Work out the finished part from the listing and answer in its coordinate system (mm). A direction names the side the tool comes from. Round coordinates to 2 decimals unless told otherwise and drop trailing zeros. Order: outer loops, then holes, each group sorted by start corner. A loop starts at its lowest first (then second) coordinate and runs counter-clockwise, first axis right, second up. Notation, with made-up numbers: M -25,80 L 8,80 A27 cw 8,113 Z; hole C -23.5,3.25 d9. An arc over 180 degrees is marked long. Return JSON: item names as keys, results as strings.
from build123d import *

# Parameters (mm, degrees)
BOSS_EXTRUDE1_DEPTH      = 10
BOSS_EXTRUDE1_DEPTH_BACK = 0.01
SKETCH1_W                = 98
SKETCH1_H                = 42
SKETCH1_R                = 6
FILLET1_R                = 5
FILLET2_R                = 5
SKETCH3_W                = 14
SKETCH3_H                = 42
BOSS_EXTRUDE4_DEPTH      = 10
SKETCH10_W               = 14
SKETCH10_H               = 42
BOSS_EXTRUDE5_DEPTH      = 10
SKETCH11_W               = 14
SKETCH11_H               = 42
BOSS_EXTRUDE6_DEPTH      = 42
FILLET3_RADIUS           = 21
FILLET3_LENGTH           = 14
CUT_EXTRUDE1_DEPTH       = 80.252760204
CUT_EXTRUDE1_DEPTH_BACK  = 80.252760204
SKETCH12_R               = 10


with BuildPart() as part:
    # Sketch1 → Boss-Extrude1 (new, two sides: drawn at the far end of the back side and taken through both)
    with BuildSketch(Plane(origin=(0, 0, 0), x_dir=(1, 0, 0), z_dir=(0, 1, 0)).offset(-BOSS_EXTRUDE1_DEPTH_BACK)):
        Rectangle(SKETCH1_W, SKETCH1_H)
        with Locations(Location((25, 0, 0), (0, 0, 270))):
            Circle(SKETCH1_R, mode=Mode.SUBTRACT)
        with Locations(Location((-25, 0, 0), (0, 0, 270))):
            Circle(SKETCH1_R, mode=Mode.SUBTRACT)
    extrude(amount=BOSS_EXTRUDE1_DEPTH + BOSS_EXTRUDE1_DEPTH_BACK)

    # Fillet1
    fillet1_edges = [part.edges().sort_by_distance(p)[0] for p in [
        (-49, 10, 0),
    ]]
    fillet(fillet1_edges, radius=FILLET1_R)

    # Fillet2
    fillet2_edges = [part.edges().sort_by_distance(p)[0] for p in [
        (49, 10, 0),
    ]]
    fillet(fillet2_edges, radius=FILLET2_R)

    # Sketch3 → Boss-Extrude4 (add)
    with BuildSketch(Plane.XZ.offset(0.01)):
        with Locations((-42, 0)):
            Rectangle(SKETCH3_W, SKETCH3_H)
    extrude(amount=BOSS_EXTRUDE4_DEPTH)

    # Sketch10 → Boss-Extrude5 (add)
    with BuildSketch(Plane.XZ.offset(0.01)):
        with Locations((42, 0)):
            Rectangle(SKETCH10_W, SKETCH10_H)
    extrude(amount=BOSS_EXTRUDE5_DEPTH)

    # Sketch11 → Boss-Extrude6 (add)
    with BuildSketch(Plane(origin=(0, 10, 0), x_dir=(1, 0, 0), z_dir=(0, 1, 0))):
        Rectangle(SKETCH11_W, SKETCH11_H)
    extrude(amount=BOSS_EXTRUDE6_DEPTH)

    # Fillet3: full round fillet: the end face becomes a half cylinder, R = half its width
    fillet3_face = Plane((0, 52, 0), x_dir=(1, 0, 0), z_dir=(0, 1, 0))  # on the end face: x along it, z out of the body
    fillet3_slab = fillet3_face.offset(-FILLET3_RADIUS / 2) * Box(FILLET3_LENGTH, 2 * FILLET3_RADIUS, FILLET3_RADIUS, mode=Mode.PRIVATE)  # the body's end, R deep
    fillet3_round = Plane((0, 31, 0), x_dir=(0, 1, 0), z_dir=(1, 0, 0)) * Cylinder(FILLET3_RADIUS, FILLET3_LENGTH, mode=Mode.PRIVATE)  # its axis R under the face
    add(fillet3_slab - fillet3_round, mode=Mode.SUBTRACT)

    # Sketch12 → Cut-Extrude1 (cut, two sides: drawn at the far end of the back side and taken through both)
    with BuildSketch(Plane(origin=(7, 0, 0), x_dir=(0, 0, -1), z_dir=(1, 0, 0)).offset(-CUT_EXTRUDE1_DEPTH_BACK)):
        with Locations((0, 31)):
            Circle(SKETCH12_R)
    extrude(amount=CUT_EXTRUDE1_DEPTH + CUT_EXTRUDE1_DEPTH_BACK, mode=Mode.SUBTRACT)


solid = part.part
Item 1: Which of the six approach directions +Z, -Z, +X, -X, +Y, -Y give full straight-line access (tool end or side, diameter ignored) to faces 4 (the flat face through (29, 10, -5)), 5 (the flat face through (-30, 10, -5)), 6 (the flat face through (49, -2, 0)), 7 (the flat face through (0, -0.01, 0))?
Output:
{"face 4": "+Z, -Z, +X, +Y", "face 5": "+Z, -Z, -X, +Y", "face 6": "+Z, -Z, +X, +Y, -Y", "face 7": "+Z, -Z, -Y"}
Item 2: Find section C-C (y = 33.5). Determine the outline of the cut face in (x, z).
Output:
{"outline": "M -7,-20.85 L 7,-20.85 L 7,-9.68 L -7,-9.68 Z; M -7,9.68 L 7,9.68 L 7,20.85 L -7,20.85 Z"}
Item 3: Find section B-B (z = 0). Determine the outline of the cut face in (x, y), plus the area to 3 significant figures.
Output:
{"outline": "M -49,-10.01 L -35,-10.01 L -35,-0.01 L -31,-0.01 L -31,10 L -44,10 A5 ccw -49,5 Z; M -19,-0.01 L 19,-0.01 L 19,10 L 7,10 L 7,21 L -7,21 L -7,10 L -19,10 Z; M -7,41 L 7,41 L 7,52 L -7,52 Z; M 31,-0.01 L 35,-0.01 L 35,-10.01 L 49,-10.01 L 49,5 A5 ccw 44,10 L 31,10 Z", "area": "1,320 mm^2"}
Item 4: Find section D-D (x = -1). Determine the outline of the cut face in (y, z), plus the area to 3 significant figures.
Output:
{"outline": "M -0.01,-21 L 31,-21 A21 ccw 31,21 L -0.01,21 Z; hole C 31,0 d20", "area": "1,680 mm^2"}
Item 5: The mould has two halves that part along Z. Classify faces 1 (the flat face through (-35, -5, 0)), 2 (the cylindrical face through (0, 52, 0)), 3 (the cylindrical face through (-30.323, 4.925, 2.769)): pulls with the +Z half, pulls with the -Z half, needs draft (parallel to the pull), parting line crosses it, or undercut.
Output:
{"face 1": "needs draft", "face 2": "parting line crosses it", "face 3": "undercut"}
Item 6: Consider line 1 along X through (y, z) = (2.5, 0); line 2 along Z through (x, y) = (-2, 31); line 3 along X through (y, z) = (-2, 3). Determine where each line is inside the solid, lowest interval first. Write a range as [from, to].
Output:
{"line 1": "x = [-49, -31], [-19, 19], [31, 49]", "line 2": "z = [-21, -10], [10, 21]", "line 3": "x = [-49, -35], [35, 49]"}
Item 7: Each of these flat-tipped pins is pushed along its axis until it touches: pin 1 (14 mm diameter, centred on x = -25, z = 0, fed in from +Y); pin 2 (4 mm diameter, centred on x = -26.5, z = -10, fed in from -Y); pin 3 (2 mm diameter, centred on x = 0, z = -4.5, fed in from +Y); pin 4 (2 mm diameter, centred on y = 38.5, z = -3, fed in from -X). Where does it stop, or does it pass through?
Output:
{"pin 1": "stops at y = 10", "pin 2": "stops at y = -0.01", "pin 3": "stops at y = 51.71", "pin 4": "passes through"}
Item 8: Find section A-A (x = -25). Determine the outline of the cut face in (y, z).
Output:
{"outline": "M -0.01,-21 L 10,-21 L 10,-6 L -0.01,-6 Z; M -0.01,6 L 10,6 L 10,21 L -0.01,21 Z"}
